The drawing under review shows one solid part. Ordinate dimensions are in mm from its lowest x, y, z. Coordinates: 2 decimals unless noted, no trailing zeros. Order: outer loops, then holes, each group sorted by start corner. A loop starts at its lowest first (then second) coordinate and runs counter-clockwise, first axis right, second up. Notation, with made-up numbers: (-30.75, 11) - (28.25, 11) arc R19 ccw to (28.25, 36) - close; hole circle Ø2 at (-22, 13.25). An arc over 180 degrees is marked (long way). Write item = value, one per line. Start each with the question number.
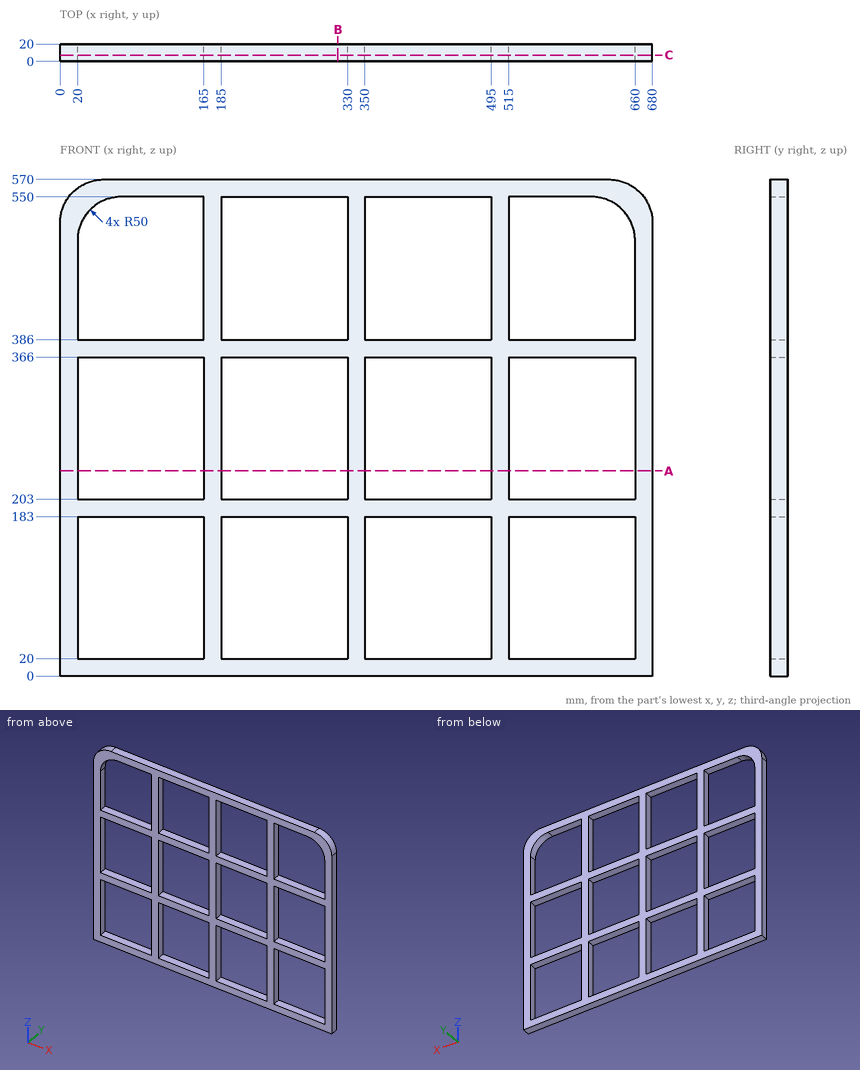
Item 1: For line 1 (Z direction, x = 579.5, y = 2.25); line 2 (X direction, y = 17.5, z = 455.5); line 3 (Z direction, x = 625, y = 15.5), list the stretches that pass through material, from the lowest coordinate up.
Item 2: Add section B-B on x = 319. Give the boundary of the cut face in (y, z).
Item 3: Add section C-C on y = 7.25. State how many separate pieces and enclosed holes the cut face has, plus the area to 3 significant figures.
Item 4: Add section A-A on z = 235.5. Give the boundary of the cut face in (x, y).
Item 5: For P1, Ø1, axis at y = 7, z = 263.5, coming from the -X side, flat-tipped, find the tip position at first contact; note if it passes through.
Worked out:
q1.line_1 = 0 to 20, 183 to 203, 366 to 386, 550 to 570
q1.line_2 = 0 to 20, 165 to 185, 330 to 350, 495 to 515, 660 to 680
q1.line_3 = 0 to 20, 183 to 203, 366 to 386, 547.7 to 570
q2.outline = (0, 0) - (20, 0) - (20, 20) - (0, 20) - close; (0, 183) - (20, 183) - (20, 203) - (0, 203) - close; (0, 366) - (20, 366) - (20, 386) - (0, 386) - close; (0, 550) - (20, 550) - (20, 570) - (0, 570) - close
q3.separate_pieces = 1
q3.enclosed_holes = 12
q3.area = 103,000 mm2
q4.outline = (0, 0) - (20, 0) - (20, 20) - (0, 20) - close; (165, 0) - (185, 0) - (185, 20) - (165, 20) - close; (330, 0) - (350, 0) - (350, 20) - (330, 20) - close; (495, 0) - (515, 0) - (515, 20) - (495, 20) - close; (660, 0) - (680, 0) - (680, 20) - (660, 20) - close
q5.P1 = 0
